from build123d import *

# Parameters (mm, degrees)
F0_W     = 60
F0_H     = 60
F1_DEPTH = 10.1
F2_R     = 3
F4_DEPTH = 45
F5_R     = 10
F6_DEPTH = 10.1


with BuildPart() as f1:
    # F0 (on Top) → F1 (new body)
    with BuildSketch(Plane.XY):
        Rectangle(F0_W, F0_H)
    extrude(amount=F1_DEPTH)

    # F2
    f2_edges = [f1.edges().sort_by_distance(p)[0] for p in [
        (30, -30, 5.05),
        (30, 30, 5.05),
        (-30, -30, 5.05),
        (-30, 30, 5.05),
    ]]
    fillet(f2_edges, radius=F2_R)

    # F3 (on face) → F4 (join)
    with BuildSketch(Plane.XY.offset(10.1)):
        with BuildLine():
            Line((-17.67767, 13.435029), (-12.513625, 8.270985))
            ThreePointArc((-12.513625, 8.270985), (-13.858193, 5.740251), (-14.696938, 3))
            Line((-14.696938, 3), (-22, 3))
            ThreePointArc((-22, 3), (-24.12132, 2.12132), (-25, 0))
            ThreePointArc((-25, 0), (-24.12132, -2.12132), (-22, -3))
            Line((-22, -3), (-14.696938, -3))
            ThreePointArc((-14.696938, -3), (-13.858193, -5.740251), (-12.513625, -8.270985))
            Line((-12.513625, -8.270985), (-17.67767, -13.435029))
            Line((-17.67767, -13.435029), (-18.73833, -12.374369))
            ThreePointArc((-18.73833, -12.374369), (-19.79899, -11.935029), (-20.85965, -12.374369))
            ThreePointArc((-20.85965, -12.374369), (-21.29899, -13.435029), (-20.85965, -14.495689))
            Line((-20.85965, -14.495689), (-17.67767, -17.67767))
            Line((-17.67767, -17.67767), (-14.495689, -20.85965))
            ThreePointArc((-14.495689, -20.85965), (-13.435029, -21.29899), (-12.374369, -20.85965))
            ThreePointArc((-12.374369, -20.85965), (-11.935029, -19.79899), (-12.374369, -18.73833))
            Line((-12.374369, -18.73833), (-13.435029, -17.67767))
            Line((-13.435029, -17.67767), (-8.270985, -12.513625))
            ThreePointArc((-8.270985, -12.513625), (-5.740251, -13.858193), (-3, -14.696938))
            Line((-3, -14.696938), (-3, -22))
            ThreePointArc((-3, -22), (-2.12132, -24.12132), (0, -25))
            ThreePointArc((0, -25), (2.12132, -24.12132), (3, -22))
            Line((3, -22), (3, -14.696938))
            ThreePointArc((3, -14.696938), (5.740251, -13.858193), (8.270985, -12.513625))
            Line((8.270985, -12.513625), (13.435029, -17.67767))
            Line((13.435029, -17.67767), (12.374369, -18.73833))
            ThreePointArc((12.374369, -18.73833), (11.935029, -19.79899), (12.374369, -20.85965))
            ThreePointArc((12.374369, -20.85965), (13.435029, -21.29899), (14.495689, -20.85965))
            Line((14.495689, -20.85965), (17.67767, -17.67767))
            Line((17.67767, -17.67767), (20.85965, -14.495689))
            ThreePointArc((20.85965, -14.495689), (21.29899, -13.435029), (20.85965, -12.374369))
            ThreePointArc((20.85965, -12.374369), (19.79899, -11.935029), (18.73833, -12.374369))
            Line((18.73833, -12.374369), (17.67767, -13.435029))
            Line((17.67767, -13.435029), (12.513625, -8.270985))
            ThreePointArc((12.513625, -8.270985), (13.858193, -5.740251), (14.696938, -3))
            Line((14.696938, -3), (22, -3))
            ThreePointArc((22, -3), (24.12132, -2.12132), (25, 0))
            ThreePointArc((25, 0), (24.12132, 2.12132), (22, 3))
            Line((22, 3), (14.696938, 3))
            ThreePointArc((14.696938, 3), (13.858193, 5.740251), (12.513625, 8.270985))
            Line((12.513625, 8.270985), (17.67767, 13.435029))
            Line((17.67767, 13.435029), (18.73833, 12.374369))
            ThreePointArc((18.73833, 12.374369), (19.79899, 11.935029), (20.85965, 12.374369))
            ThreePointArc((20.85965, 12.374369), (21.29899, 13.435029), (20.85965, 14.495689))
            Line((20.85965, 14.495689), (17.67767, 17.67767))
            Line((17.67767, 17.67767), (14.495689, 20.85965))
            ThreePointArc((14.495689, 20.85965), (13.435029, 21.29899), (12.374369, 20.85965))
            ThreePointArc((12.374369, 20.85965), (11.935029, 19.79899), (12.374369, 18.73833))
            Line((12.374369, 18.73833), (13.435029, 17.67767))
            Line((13.435029, 17.67767), (8.270985, 12.513625))
            ThreePointArc((8.270985, 12.513625), (5.740251, 13.858193), (3, 14.696938))
            Line((3, 14.696938), (3, 22))
            ThreePointArc((3, 22), (2.12132, 24.12132), (0, 25))
            ThreePointArc((0, 25), (-2.12132, 24.12132), (-3, 22))
            Line((-3, 22), (-3, 14.696938))
            ThreePointArc((-3, 14.696938), (-5.740251, 13.858193), (-8.270985, 12.513625))
            Line((-8.270985, 12.513625), (-13.435029, 17.67767))
            Line((-13.435029, 17.67767), (-12.374369, 18.73833))
            ThreePointArc((-12.374369, 18.73833), (-11.935029, 19.79899), (-12.374369, 20.85965))
            ThreePointArc((-12.374369, 20.85965), (-13.435029, 21.29899), (-14.495689, 20.85965))
            Line((-14.495689, 20.85965), (-17.67767, 17.67767))
            Line((-17.67767, 17.67767), (-20.85965, 14.495689))
            ThreePointArc((-20.85965, 14.495689), (-21.29899, 13.435029), (-20.85965, 12.374369))
            ThreePointArc((-20.85965, 12.374369), (-19.79899, 11.935029), (-18.73833, 12.374369))
            Line((-18.73833, 12.374369), (-17.67767, 13.435029))
        make_face()
        with BuildLine():
            ThreePointArc((-10, 0), (-9.238795, 3.826834), (-7.071068, 7.071068))
            ThreePointArc((-7.071068, 7.071068), (-3.826834, 9.238795), (0, 10))
            ThreePointArc((0, 10), (3.826834, 9.238795), (7.071068, 7.071068))
            ThreePointArc((7.071068, 7.071068), (9.238795, 3.826834), (10, 0))
            ThreePointArc((10, 0), (9.238795, -3.826834), (7.071068, -7.071068))
            ThreePointArc((7.071068, -7.071068), (3.826834, -9.238795), (0, -10))
            ThreePointArc((0, -10), (-3.826834, -9.238795), (-7.071068, -7.071068))
            ThreePointArc((-7.071068, -7.071068), (-9.238795, -3.826834), (-10, 0))
        make_face(mode=Mode.SUBTRACT)
    extrude(amount=F4_DEPTH)

    # F5 (on face) → F6 (cut, through all)
    with BuildSketch(Plane(origin=(0, 0, 0), x_dir=(1, 0, 0), z_dir=(0, 0, -1))):
        Circle(F5_R)
    extrude(amount=-F6_DEPTH, mode=Mode.SUBTRACT)


solid = f1.part
Check sheet for the modelled part. Datum: model origin and axes. Units: mm. A direction names the side the tool comes from. Round coordinates to 2 decimals unless told otherwise and drop trailing zeros. Order: outer loops, then holes, each group sorted by start corner. A loop starts at its lowest first (then second) coordinate and runs counter-clockwise, first axis right, second up. Notation, with made-up numbers: M 9.5,-3.5 L 36.5,-3.5 A20 cw 36.5,18.5 Z; hole C 0,77 d3. An arc over 180 degrees is marked long. One line per item, written item: value. Start each with the question number.
1. Section check A-A on z = 8. Enter the section's corners in (x, y), and give its area (3 significant figures).
2. Section check C-C on x = -20. Enter the section's corners in (y, z), and give its area (3 significant figures).
3. Scan lines: line 1 along X through (y, z) = (0, 4); line 2 along X through (y, z) = (19, 30); line 3 along X through (y, z) = (15.5, 45). Record each from-to range of solid material in increasing order.
4. Section check B-B on x = 6. Enter the section's corners in (y, z), and give its area (3 significant figures).
5. Gauge pin test, flat ends, axial feed: P1, Ø3.5, axis at x = 17, z = 40.5, coming from the -Y side; P2, Ø6, axis at y = 13.5, z = 36, coming from the +X side; P3, Ø6, axis at x = -15, z = 35, coming from the -Y side. Record the tip position at first contact, or that the pin passes through.
6. Access from +Z, -Z, +X, -X, +Y, -Y to the whole of each face (thin tool, end or side, straight path). Record for faces 1 (the flat face through (18, 3, 32)), 2 (the flat face through (10.89, 15.13, 32.28)), 3 (the flat face through (3, 18, 32)).
7. Release check for a two-part mould opening along X. For faces 4 (the flat face through (0, 30, 5)), 5 (the flat face through (-3, 18, 32)), 6 (the flat face through (-30, 0, 5)) record: released by +X, released by -X, zero draft, split by the parting line, or undercut.
Results found:
1. outline: M -30,-27 A3 ccw -27,-30 L 27,-30 A3 ccw 30,-27 L 30,27 A3 ccw 27,30 L -27,30 A3 ccw -30,27 Z; hole C 0,0 d20
1. area: 3,280 mm^2
2. outline: M -30,0 L 30,0 L 30,10.1 L 15.36,10.1 L 15.36,55.1 L 11.95,55.1 L 11.95,10.1 L 3,10.1 L 3,55.1 L -3,55.1 L -3,10.1 L -11.95,10.1 L -11.95,55.1 L -15.36,55.1 L -15.36,10.1 L -30,10.1 Z
2. area: 1,180 mm^2
3. line 1: -30 to -10, 10 to 30
3. line 2: -16.36 to -12.17, -3 to 3, 12.17 to 16.36
3. line 3: -19.86 to -11.26, -3 to 3, 11.26 to 19.86
4. outline: M -30,0 L -8,0 L -8,55.1 L -13.75,55.1 L -13.75,10.1 L -30,10.1 Z; M 8,0 L 30,0 L 30,10.1 L 13.75,10.1 L 13.75,55.1 L 8,55.1 Z
4. area: 962 mm^2
5. P1: y = -20.11
5. P2: x = 21.3
5. P3: y = -21.3
6. face 1: +Z, +X
6. face 2: +Z
6. face 3: +Z, +Y
7. face 4: zero draft
7. face 5: undercut
7. face 6: released by -X
